from build123d import *

# Parameters (mm, degrees)
BOSS_EXTRUDE1_DEPTH = 0.75


with BuildPart() as part:
    # Sketch1 → Revolve1 (revolve)
    with BuildSketch(Plane(origin=(0, 0, 0), x_dir=(1, 0, 0), z_dir=(0, 1, 0))):
        Polygon((3.05, 0), (0, -2), (0, -7), (3.05, -7), align=None)
    revolve(axis=Axis((4.6, 0, 0), (0, 0, 1)))

    # Sketch2 → Boss-Extrude1 (add)
    with BuildSketch(Plane.XY.offset(7)):
        with BuildLine():
            Line((0.110011136, 1), (1.6626194, 1))
            ThreePointArc((1.6626194, 1), (1.538733475, 0.506805736), (1.497065133, 0))
            ThreePointArc((1.497065133, 0), (1.538733475, -0.506805736), (1.6626194, -1))
            Line((1.6626194, -1), (0.110011136, -1))
            ThreePointArc((0.110011136, -1), (0, 0), (0.110011136, 1))
        make_face()
    extrude(amount=BOSS_EXTRUDE1_DEPTH)


solid = part.part
Can you work these out from the model? Positions are in its coordinate system, mm. Round coordinates to 2 decimals unless told otherwise and drop trailing zeros. Write each loop counter-clockwise with the first axis right and the second up, starting at its lowest first coordinate (ties: lowest second). Pieces come first, ordered by that corner, then holes. Notation, with made-up numbers: (1, 34) - (54, 34) arc R19 ccw to (54, 56) - close; hole circle Ø6 at (58, 8). An arc over 180 degrees is marked (long way). Write each question's results on one line, items separated by ' | '. Start each with the question number.
1) For pin 1 Ø0.8 at (x, z) = (0.5, 7.5) entering from -Y; pin 2 Ø1.9 at (x, y) = (4.6, 0) entering from +Z; pin 3 Ø2 at (x, z) = (3, 3) entering from -Y; pin 4 Ø0.8 at (x, z) = (1, 7.5) entering from +Y, each with a flat end and sliding along its axis, tell me the tip position at first contact or that it passes through.
2) Please list where these lines run through material, in increasing order: line 1 (X direction, y = 0, z = 2.25); line 2 (Y direction, x = 4.6, z = 5.5); line 3 (Y direction, x = 4, z = 1.25).
3) Suppose I cut it at A-A (x = 4.6). List the corners of the cut face in (y, z) for me, and give its area (3 significant figures).
4) Suppose I cut it at C-C (z = 5.75). List the corners of the cut face in (x, y) for me, and give its area (3 significant figures).
5) We'd pull the mould along Y, two halves only. Please class faces 1 (the cylindrical face through (3.122, -0.466, 3.451)), 2 (the flat face through (1, 0, 7.75)), 3 (the cylindrical face through (0, 0, 5)): released by +Y, released by -Y, zero draft, split by the parting line, or undercut.
Here are the results:
1) pin 1: stops at y = -1 | pin 2: passes through | pin 3: stops at y = -4.56 | pin 4: stops at y = 1
2) line 1: x = 0 to 3.05, 6.15 to 9.2 | line 2: y = -4.6 to -1.55, 1.55 to 4.6 | line 3: y = -3.4 to -1.43, 1.43 to 3.4
3) outline: (-4.6, 2) - (-1.55, 0) - (-1.55, 7) - (-4.6, 7) - close; (1.55, 0) - (4.6, 2) - (4.6, 7) - (1.55, 7) - close | area: 36.6 mm2
4) outline: circle Ø9.2 at (4.6, 0); hole circle Ø3.1 at (4.6, 0) | area: 58.9 mm2
5) face 1: undercut | face 2: zero draft | face 3: split by the parting line
